The model under review builds one solid part; all positions refer to its coordinate system, in mm. Face numbers are marked on the shaded views. A direction names the side the tool comes from. Give positions to 0.01 mm unless a question says otherwise; leave off trailing zeros. Write each loop counter-clockwise with the first axis right and the second up, starting at its lowest first coordinate (ties: lowest second). Pieces come first, ordered by that corner, then holes. Notation, with made-up numbers: (20.5, 22) - (61.5, 22) arc R27 cw to (61.5, 58) - close; hole circle Ø6 at (22.25, 12). An arc over 180 degrees is marked (long way). One line per question, with ' | ' between items. Start each with the question number.
```python
from build123d import *

# Parameters (mm, degrees)
F0_W     = 125
F0_H     = 75
F1_DEPTH = 35
F2_W     = 70
F2_H     = 25
F3_DEPTH = 70.001
F4_W     = 27.5
F4_H     = 15
F5_DEPTH = 75.001


with BuildPart() as f1:
    # F0 (on Front) → F1 (new body, symmetric)
    with BuildSketch(Plane.XZ):
        with Locations((62.5, 37.5)):
            Rectangle(F0_W, F0_H)
    extrude(amount=F1_DEPTH, both=True)

    # F2 (on face) → F3 (cut, through all)
    with BuildSketch(Plane.XZ.offset(35)):
        with Locations((60, 62.5)):
            Rectangle(F2_W, F2_H)
    extrude(amount=-F3_DEPTH, mode=Mode.SUBTRACT)

    # F4 (on face) → F5 (cut, through all)
    with BuildSketch(Plane.XY.offset(75)):
        Polygon((0, -5), (0, -35), (105, -35), (105, -5), (70, -5), (42.5, -5), align=None)
        with Locations((56.25, 2.5)):
            Rectangle(F4_W, F4_H)
    extrude(amount=-F5_DEPTH, mode=Mode.SUBTRACT)


solid = f1.part
```
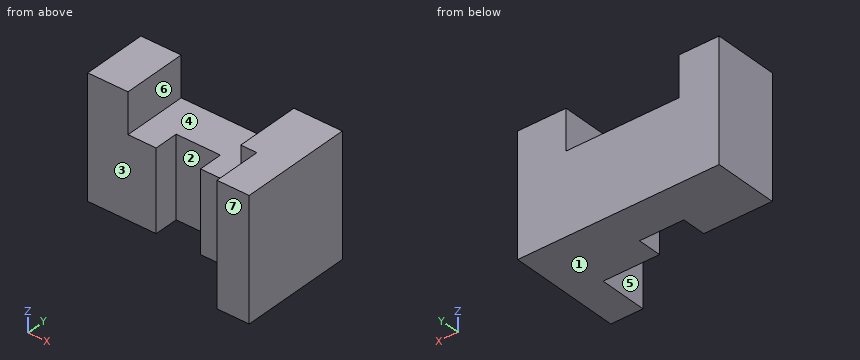
Item 1: Clearance check with flat-ended pins moving along their axes: P1, Ø1, axis at x = 44, y = 17.5, coming from the +Z side; P2, Ø1.5, axis at x = 15, z = 59, coming from the -Y side; P3, Ø9, axis at y = -19, z = 26.5, coming from the -X side. State where each tip first meets the part, or that it passes through.
Item 2: The part is to be moulded in two halves that separate along X. For the marked faces 5, 6 and 7, say which applies: +X half, -X half, draft (parallel to the pull), parting line (faces both ways), or undercut.
Item 3: Machinability: for the marked faces 1, 2, 3 and 4, which of the approach directions +Z, -Z, +X, -X, +Y, -Y give a long, thin tool a straight path to every point of the face, cutting with its end or side? Answer none if there is none.
Item 4: For probe 1 along X at (y, z) = (1.5, 64.5); probe 2 along X at (y, z) = (6, 17); probe 3 along Y at (x, z) = (13, 38), list the stretches that pass through material, from the lowest coordinate up.
Item 5: Take a section at C-C (y = 14.5). Give the boundary of the cut face in (x, z).
Item 6: Take a section at D-D (z = 30.5). Give the boundary of the cut face in (x, y).
Item 7: Take a section at B-B (y = 3). Give the boundary of the cut face in (x, z), plus the area to 3 significant figures.
Item 8: Take a section at A-A (z = 59). Give the boundary of the cut face in (x, y), plus the area to 3 significant figures.
Check sheet entries:
1) P1: stops at z = 50 | P2: stops at y = -5 | P3: stops at x = 105
2) face 5: -X half | face 6: undercut | face 7: draft
3) face 1: -Z, +X, -X, +Y, -Y | face 2: +Z, -Z, -Y | face 3: +Z, -Z, -X, -Y | face 4: +Z, +Y, -Y
4) probe 1: x = 0 to 25, 95 to 125 | probe 2: x = 0 to 42.5, 70 to 125 | probe 3: y = -5 to 35
5) outline: (0, 0) - (125, 0) - (125, 75) - (95, 75) - (95, 50) - (25, 50) - (25, 75) - (0, 75) - close
6) outline: (0, -5) - (42.5, -5) - (42.5, 10) - (70, 10) - (70, -5) - (105, -5) - (105, -35) - (125, -35) - (125, 35) - (0, 35) - close
7) outline: (0, 0) - (42.5, 0) - (42.5, 50) - (25, 50) - (25, 75) - (0, 75) - close; (70, 0) - (125, 0) - (125, 75) - (95, 75) - (95, 50) - (70, 50) - close | area: 6,250 mm^2
8) outline: (0, -5) - (25, -5) - (25, 35) - (0, 35) - close; (95, -5) - (105, -5) - (105, -35) - (125, -35) - (125, 35) - (95, 35) - close | area: 2,800 mm^2
